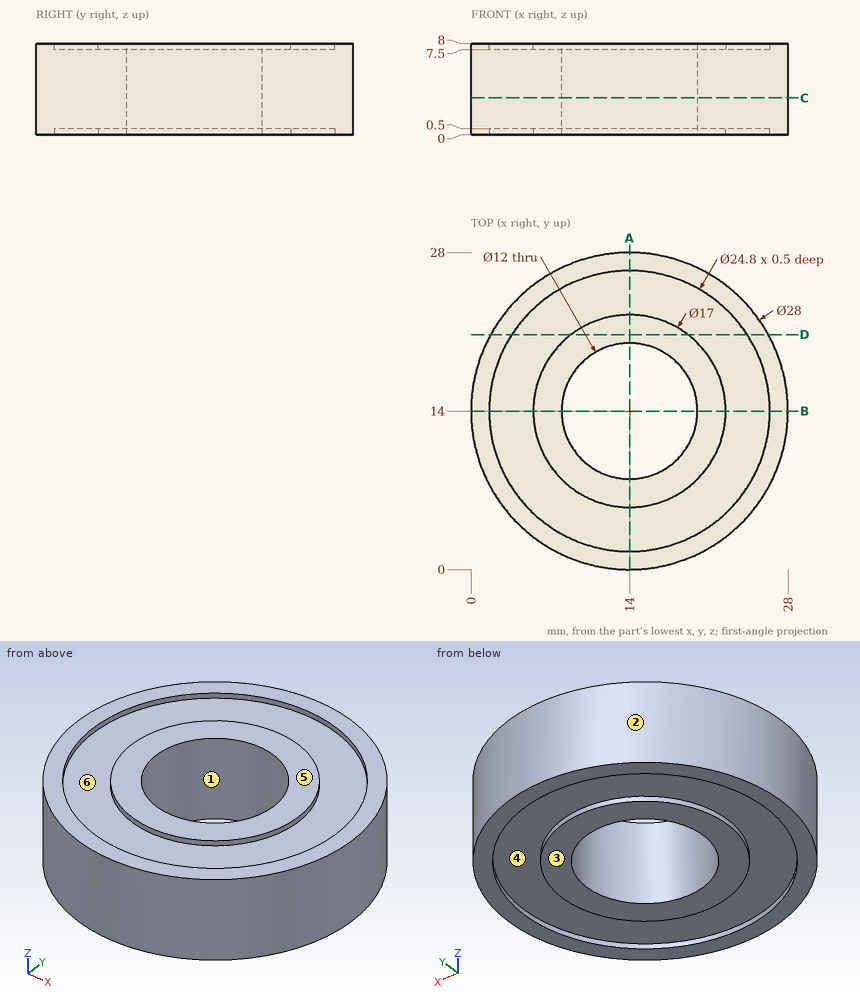
Verification items for this drawing (mm, ordinates from the low corner). A direction names the side the tool comes from. Give positions to 0.01 mm unless a question says otherwise; leave off trailing zeros. Write each loop counter-clockwise with the first axis right and the second up, starting at its lowest first coordinate (ties: lowest second). Pieces come first, ordered by that corner, then holes.
1) Go/stop test with flat-tipped pins: pin 1 Ø4 at (x, z) = (21, 2.5) entering from +Y; pin 2 Ø3 at (x, z) = (24, 7) entering from -Y; pin 3 Ø2 at (y, z) = (22, 5) entering from -X. Record where each tip stops, or that it passes through.
Values follow:
pin 1: stops at y = 27.08
pin 2: stops at y = 2.88
pin 3: stops at x = 1.88
2) Set-up check for the marked faces 4, 5 and 6: record each of +Z, -Z, +X, -X, +Y, -Y from which the full face is reachable in a straight line by a thin tool's end or side.
Values follow:
face 4: -Z
face 5: +Z, +X, -X, +Y, -Y
face 6: +Z
3) Cross-section at C-C (z = 3.25). Record the boundary of the cut face in (x, y), plus the area to 3 significant figures.
Values follow:
outline: circle Ø28 at (14, 14); hole circle Ø12 at (14, 14)
area: 503 mm2
4) Release check for a two-part mould opening along Y. For the marked faces 1, 2 and 3 record: released by +Y, released by -Y, zero draft, split by the parting line, or undercut.
Values follow:
face 1: undercut
face 2: split by the parting line
face 3: zero draft
5) Thickness scan on line 1 (Y direction, x = 14, z = 0.35); line 2 (Y direction, x = 14, z = 5.75); line 3 (X direction, y = 17, z = 3.25). Record the ranges inside material, lowest first.
Values follow:
line 1: y = 0 to 1.6, 5.5 to 8, 20 to 22.5, 26.4 to 28
line 2: y = 0 to 8, 20 to 28
line 3: x = 0.33 to 8.8, 19.2 to 27.67
6) Cross-section at A-A (x = 14). Record the boundary of the cut face in (y, z).
Values follow:
outline: (0, 0) - (1.6, 0) - (1.6, 0.5) - (5.5, 0.5) - (5.5, 0) - (8, 0) - (8, 8) - (5.5, 8) - (5.5, 7.5) - (1.6, 7.5) - (1.6, 8) - (0, 8) - close; (20, 0) - (22.5, 0) - (22.5, 0.5) - (26.4, 0.5) - (26.4, 0) - (28, 0) - (28, 8) - (26.4, 8) - (26.4, 7.5) - (22.5, 7.5) - (22.5, 8) - (20, 8) - close
7) Cross-section at D-D (y = 20.75). Record the boundary of the cut face in (x, z), plus the area to 3 significant figures.
Values follow:
outline: (1.73, 0) - (3.6, 0) - (3.6, 0.5) - (8.83, 0.5) - (8.83, 0) - (19.17, 0) - (19.17, 0.5) - (24.4, 0.5) - (24.4, 0) - (26.27, 0) - (26.27, 8) - (24.4, 8) - (24.4, 7.5) - (19.17, 7.5) - (19.17, 8) - (8.83, 8) - (8.83, 7.5) - (3.6, 7.5) - (3.6, 8) - (1.73, 8) - close
area: 186 mm2
